```python
from build123d import *

# Parameters (mm, degrees)
BOSS_EXTRUDE1_DEPTH      = 5
BOSS_EXTRUDE1_DEPTH_BACK = 563.8
CUT_EXTRUDE1_DEPTH       = 7.42512
BOSS_EXTRUDE2_DEPTH      = 91.3
SKETCH4_R                = 0.69
SKETCH4_R_2              = 0.51
CUT_EXTRUDE2_DEPTH       = 2


with BuildPart() as part:
    # Sketch1 → Boss-Extrude1 (new body, two sides)
    with BuildSketch(Plane(origin=(0, 0, 0), x_dir=(0, 0, -1), z_dir=(1, 0, 0))) as boss_extrude1_sk:
        with BuildLine():
            Line((0, 0), (-61, 0))
            ThreePointArc((-61, 0), (-64.21256, -3.21256), (-61, -6.42512))
            Line((-61, -6.42512), (0, -6.42512))
            Line((0, -6.42512), (5, -6.42512))
            Line((5, -6.42512), (5, -6.26256))
            Line((5, -6.26256), (-61, -6.26256))
            ThreePointArc((-61, -6.26256), (-64.05, -3.21256), (-61, -0.16256))
            Line((-61, -0.16256), (5, -0.16256))
            Line((5, -0.16256), (5, 0))
            Line((5, 0), (0, 0))
        make_face()
    extrude(amount=BOSS_EXTRUDE1_DEPTH)
    extrude(boss_extrude1_sk.sketch, amount=-BOSS_EXTRUDE1_DEPTH_BACK)

    # Sketch2 → Cut-Extrude1 (cut, through all)
    with BuildSketch(Plane(origin=(0, 0, 0), x_dir=(1, 0, 0), z_dir=(0, 1, 0))):
        with BuildLine():
            Line((5, 0), (1, 0))
            ThreePointArc((1, 0), (0.292893219, 0.292893219), (0, 1))
            Line((0, 1), (0, 5))
            Line((0, 5), (-5, 5))
            Line((-5, 5), (-5, 1))
            ThreePointArc((-5, 1), (-5.292893219, 0.292893219), (-6, 0))
            Line((-6, 0), (-457.8, 0))
            ThreePointArc((-457.8, 0), (-458.507106781, 0.292893219), (-458.8, 1))
            Line((-458.8, 1), (-458.8, 5))
            Line((-458.8, 5), (-463.8, 5))
            Line((-463.8, 5), (-463.8, 1))
            ThreePointArc((-463.8, 1), (-464.092893219, 0.292893219), (-464.8, 0))
            Line((-464.8, 0), (-563.8, 0))
            Line((-563.8, 0), (-563.8, 10))
            Line((-563.8, 10), (5, 10))
            Line((5, 10), (5, 0))
        make_face()
    extrude(amount=-CUT_EXTRUDE1_DEPTH, mode=Mode.SUBTRACT)

    # Sketch3 → Boss-Extrude2 (add)
    with BuildSketch(Plane.ZY.offset(563.8)):
        with BuildLine():
            Line((61, -0.23114), (0, -0.23114))
            Line((0, -0.23114), (0, 0))
            Line((0, 0), (61, 0))
            ThreePointArc((61, 0), (64.21256, -3.21256), (61, -6.42512))
            Line((61, -6.42512), (0, -6.42512))
            Line((0, -6.42512), (0, -6.19398))
            Line((0, -6.19398), (61, -6.19398))
            ThreePointArc((61, -6.19398), (63.98142, -3.21256), (61, -0.23114))
        make_face()
    extrude(amount=-BOSS_EXTRUDE2_DEPTH)

    # Sketch4 → Cut-Extrude2 (cut)
    with BuildSketch(Plane(origin=(0, 0, 0), x_dir=(1, 0, 0), z_dir=(0, 1, 0))):
        with Locations(Location((-560.001, -43.918, 0), (0, 0, 270))):  # turned: the seam where the file's is
            Circle(SKETCH4_R)
        with Locations(Location((-534.001, -43.918, 0), (0, 0, 270))):  # turned: the seam where the file's is
            Circle(SKETCH4_R_2)
        with Locations(Location((-531.001, -50.418, 0), (0, 0, 270))):  # turned: the seam where the file's is
            Circle(SKETCH4_R)
        with Locations(Location((-505.001, -50.418, 0), (0, 0, 270))):  # turned: the seam where the file's is
            Circle(SKETCH4_R_2)
        with Locations(Location((-502.001, -56.918, 0), (0, 0, 270))):  # turned: the seam where the file's is
            Circle(SKETCH4_R)
        with Locations(Location((-476.001, -56.918, 0), (0, 0, 270))):  # turned: the seam where the file's is
            Circle(SKETCH4_R_2)
    extrude(amount=-CUT_EXTRUDE2_DEPTH, mode=Mode.SUBTRACT)


solid = part.part
```
Geometry: final body of the model. Coordinates: model frame, mm. Round coordinates to 2 decimals unless told otherwise and drop trailing zeros. Order: outer loops, then holes, each group sorted by start corner. A loop starts at its lowest first (then second) coordinate and runs counter-clockwise, first axis right, second up. Notation, with made-up numbers: (-2.75, 50) -> (18.25, 50) arc R12 cw to (18.25, 54) -> close; hole circle Ø4 at (5, -31). An arc over 180 degrees is marked (long way). Use one line per item in the form item = value.
(1) Ray query, probe 1 along Y at (x, z) = (-197.5, 23); probe 2 along Z at (x, y) = (-352.5, -2.5); probe 3 along Z at (x, y) = (-221, -4). Return the intervals inside material, ascending. Write a range as [from, to].
Results list:
probe_1 = [-6.43, -6.26], [-0.16, 0]
probe_2 = [63.97, 64.13]
probe_3 = [63.95, 64.11]
(2) Section B-B on x = -390.5. Return loops of the section in (y, z).
Results list:
outline = (-6.43, 0) -> (-6.26, 0) -> (-6.26, 61) arc R3.05 cw to (-0.16, 61) -> (-0.16, 0) -> (0, 0) -> (0, 61) arc R3.21 ccw to (-6.43, 61) -> close
(3) Draft query along Y for faces 1 (the face through (-275, 0, 35)), 2 (the face through (-519, -0.231, 31)), 3 (the face through (-275, -6.425, 36)). Return one class per face: pulls with the +Y half, pulls with the -Y half, needs draft (parallel to the pull), parting line crosses it, or undercut.
Results list:
face_1 = pulls with the +Y half
face_2 = undercut
face_3 = pulls with the -Y half
(4) Section A-A on z = 10.5. Return loops of the section in (x, y), and give its area (3 significant figures).
Results list:
outline = (-563.8, -6.43) -> (5, -6.43) -> (5, -6.26) -> (-472.5, -6.26) -> (-472.5, -6.19) -> (-563.8, -6.19) -> close; (-563.8, -0.23) -> (-472.5, -0.23) -> (-472.5, -0.16) -> (5, -0.16) -> (5, 0) -> (-563.8, 0) -> close
area = 197 mm^2
(5) First-contact query: pin 1 Ø0.8 at (x, z) = (-476.001, 56.918) entering from +Y; pin 2 Ø3 at (x, y) = (-412.5, -2.5) entering from -Z; pin 3 Ø1 at (x, y) = (-215, -3) entering from -Z. Flat tips, straight axial feed; report the tip coordinate or a pass-through.
Results list:
pin_1 = -6.19
pin_2 = 63.1
pin_3 = 63.97
